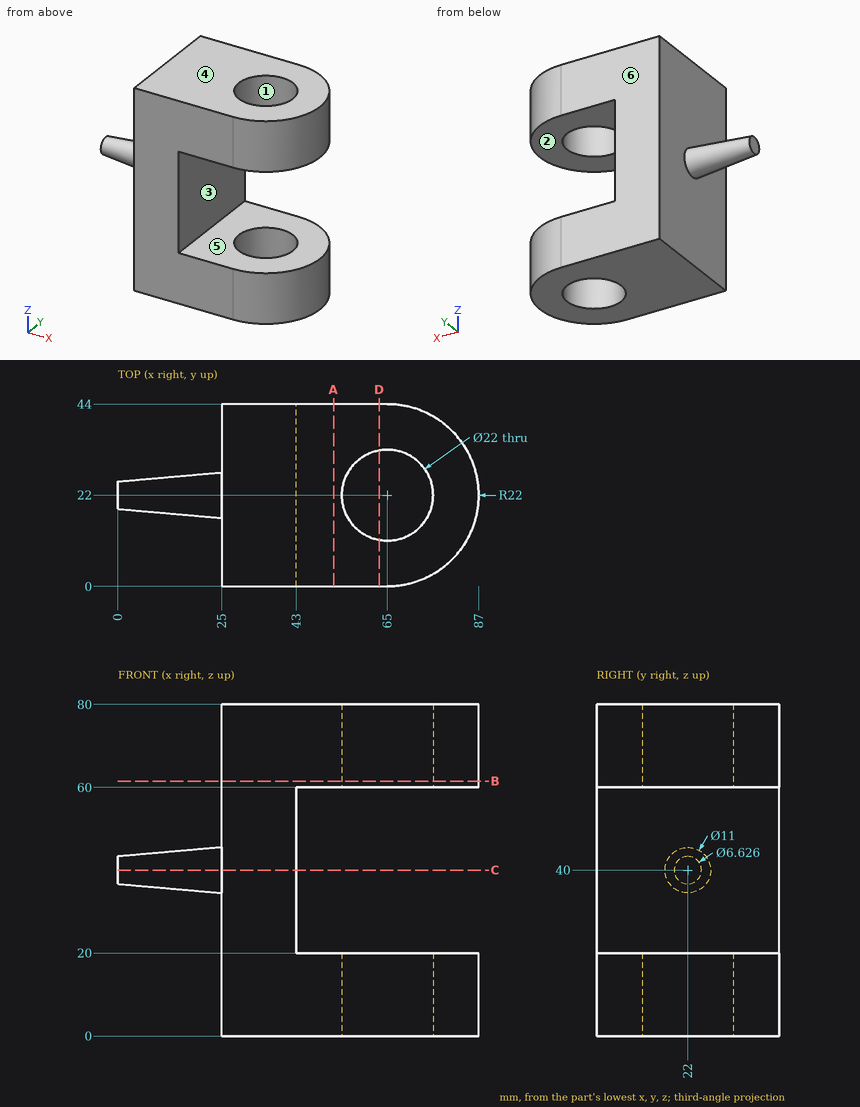
Can you work these out from the drawing? Everything is in mm from the part's minimum corner. A direction names the side the tool comes from. Round coordinates to 2 decimals unless told otherwise and drop trailing zeros. Order: outer loops, then holes, each group sorted by start corner. A loop starts at its lowest first (then second) coordinate and runs counter-clockwise, first axis right, second up. Notation, with made-up numbers: (-27, -14.75) -> (-9, -14.75) arc R16 cw to (-9, 12.25) -> close; hole circle Ø7 at (6.25, 88). An arc over 180 degrees is marked (long way). Return JSON: item names as keys, results as strings. Group by question number.
1. If we section it at D-D, the plane x = 63: Write out the boundary of the cut face in (y, z).
2. If we section it at C-C, the plane z = 40: Write out the boundary of the cut face in (x, y), then the cut area to 3 significant figures.
3. Will these pins go through, and if not, where does the flat tip stop? pin 1 (17.5 mm diameter, centred on x = 65, y = 22, fed in from -Z); pin 2 (4 mm diameter, centred on x = 72, z = 69.5, fed in from -Y) (1 decimal); pin 3 (12 mm diameter, centred on y = 15, z = 30, fed in from +X); pin 4 (4 mm diameter, centred on y = 20, z = 10.5, fed in from -X).
4. If we section it at B-B, the plane z = 61.5: Write out the boundary of the cut face in (x, y).
5. Which directions (+Z, -Z, +X, -X, +Y, -Y) give clear straight access to the entire face, cutting with the end or side of a thin tool? Please do the marked faces 1 and 2.
6. If we section it at A-A, the plane x = 52: Write out the boundary of the cut face in (y, z), then the cut area to 3 significant figures.
7. We'd pull the mould along Z, two halves only. Please class the marked faces 3, 4, 5 and 6: released by +Z, released by -Z, zero draft, split by the parting line, or undercut.
8. I need wall thicknesses on line 1 (Z direction, x = 43.5, y = 17); line 2 (X direction, y = 22, z = 7); line 3 (X direction, y = 29, z = 74.5) (1 decimal). Which ranges of each line are inside material? Lowest first, please. Write a range as [from, to].
Output values:
{
 "1": {"outline": "(0, 0) -> (11.18, 0) -> (11.18, 20) -> (0, 20) -> close; (0, 60) -> (11.18, 60) -> (11.18, 80) -> (0, 80) -> close; (32.82, 0) -> (44, 0) -> (44, 20) -> (32.82, 20) -> close; (32.82, 60) -> (44, 60) -> (44, 80) -> (32.82, 80) -> close"},
 "2": {"outline": "(0, 18.69) -> (25, 16.5) -> (25, 0) -> (43, 0) -> (43, 44) -> (25, 44) -> (25, 27.5) -> (0, 25.31) -> close", "area": "1,010 mm²"},
 "3": {"pin 1": "through", "pin 2": "y = 0.6", "pin 3": "x = 43", "pin 4": "x = 25"},
 "4": {"outline": "(25, 0) -> (65, 0) arc R22 ccw to (65, 44) -> (25, 44) -> close; hole circle Ø22 at (65, 22)"},
 "5": {"face 1": "+Z, -Z", "face 2": "+X, +Y, -Y"},
 "6": {"outline": "(0, 0) -> (44, 0) -> (44, 20) -> (0, 20) -> close; (0, 60) -> (44, 60) -> (44, 80) -> (0, 80) -> close", "area": "1,760 mm²"},
 "7": {"face 3": "undercut", "face 4": "released by +Z", "face 5": "undercut", "face 6": "zero draft"},
 "8": {"line 1": "[0, 20], [60, 80]", "line 2": "[25, 54], [76, 87]", "line 3": "[25, 56.5], [73.5, 85.9]"}
}
